```python
from build123d import *

# Parameters (mm, degrees)
BOSS_EXTRUDE1_DEPTH     = 20
CUT_EXTRUDE1_DEPTH      = 97.932966679
CUT_EXTRUDE1_DEPTH_BACK = 97.932966679
CUT_EXTRUDE3_DEPTH      = 97.932966679


with BuildPart() as part:
    # Sketch2 → Boss-Extrude1 (new body)
    with BuildSketch(Plane.XY):
        Polygon((16, 16), (16, -16), (-16, -16), (-16, -11), (-11, -11), (11, -11), (11, 11), (-11, 11), (-11, 9), (-16, 14), (-16, 16), align=None)
    extrude(amount=BOSS_EXTRUDE1_DEPTH)

    # Sketch3 → Loft1 section 0
    with BuildSketch(Plane.XZ.offset(16)):
        with BuildLine():
            Line((-16, 0), (16, 0))
            Line((16, 0), (16, 20))
            Line((16, 20), (-16, 20))
            Line((-16, 20), (-16, 0))
        make_face()
    # Sketch4 → Loft1 section 1
    with BuildSketch(Plane(origin=(0, -86, 0), x_dir=(-1, 0, 0), z_dir=(0, -1, 0))):
        with BuildLine():
            Line((40, 0), (-40, 0))
            Line((-40, 0), (-40, -20))
            Line((-40, -20), (40, -20))
            Line((40, -20), (40, 0))
        make_face()
    loft()

    # Sketch5 → Cut-Extrude1 (cut, two sides: drawn at the far end of the back side and taken through both)
    with BuildSketch(Plane(origin=(0, 0, 0), x_dir=(0, 0, -1), z_dir=(1, 0, 0)).offset(-CUT_EXTRUDE1_DEPTH_BACK)):
        Polygon((0, -81), (-15, -81), (-15, -64), (0, -21), align=None)
    extrude(amount=CUT_EXTRUDE1_DEPTH + CUT_EXTRUDE1_DEPTH_BACK, mode=Mode.SUBTRACT)

    # Sketch6 → Cut-Extrude3 (cut, through all)
    with BuildSketch(Plane.XY):
        Polygon((-1.810810811, -20.864864865), (1.810810811, -20.864864865), (19, -71), (-19, -71), align=None)
    extrude(amount=CUT_EXTRUDE3_DEPTH, mode=Mode.SUBTRACT)


solid = part.part
```
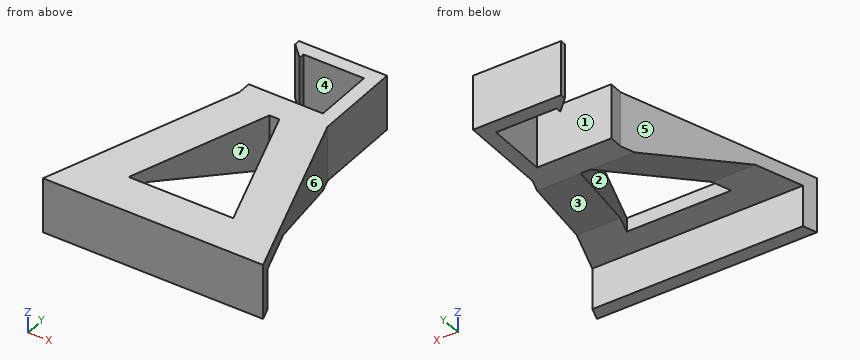
Design review of the part built by this model. Coordinates are the model's own, in mm. Face numbers are marked on the shaded views. A direction names the side the tool comes from. Give positions to 0.01 mm unless a question says otherwise; leave off trailing zeros. Write each loop counter-clockwise with the first axis right and the second up, starting at its lowest first coordinate (ties: lowest second). Pieces come first, ordered by that corner, then holes. Notation, with made-up numbers: (-34.5, -2) -> (-2.5, -2) arc R19 ccw to (-2.5, 8) -> close; hole circle Ø2 at (-39, 20.5). An arc over 180 degrees is marked (long way). Answer in a Markdown table with one row per item.
(1) Mouldability with a two-part tool opening along X and no side actions: class the marked faces 4, 5, 6 and 7 as +X half, -X half, draft (parallel to the pull), parting line (faces both ways), or undercut.
Results:
| item | result |
|---|---|
| face 4 | undercut |
| face 5 | -X half |
| face 6 | +X half |
| face 7 | undercut |
(2) Consider section A-A (z = 13.5). State the section outline as (x, y) points.
Results:
| item | result |
|---|---|
| outline | (-40, -86) -> (40, -86) -> (38.29, -81) -> (-38.29, -81) -> close; (-30.98, -59.7) -> (-15.13, -59.7) -> (-1.81, -20.86) -> (1.81, -20.86) -> (15.13, -59.7) -> (30.98, -59.7) -> (16, -16) -> (16, 16) -> (-16, 16) -> (-16, 14) -> (-11, 9) -> (-11, 11) -> (11, 11) -> (11, -11) -> (-16, -11) -> (-16, -16) -> close |
(3) Consider section D-D (x = -6.5). State the section outline as (y, z) points, then the cut area to 3 significant figures.
Results:
| item | result |
|---|---|
| outline | (-86, 0) -> (-81, 0) -> (-81, 15) -> (-71, 15) -> (-71, 20) -> (-86, 20) -> close; (-34.54, 4.72) -> (-21, 0) -> (-11, 0) -> (-11, 20) -> (-34.54, 20) -> close; (11, 0) -> (16, 0) -> (16, 20) -> (11, 20) -> close |
| area | 689 mm2 |
(4) For the marked faces 1, 2 and 3, list the 3-axis set-ups (+Z, -Z, +X, -X, +Y, -Y) from which the entire face can be reached by the end or side of a thin tool; tool diameter is ignored.
Results:
| item | result |
|---|---|
| face 1 | +Z, -Z, -X |
| face 2 | +Z, -Z |
| face 3 | -Z, +X, -X |
(5) Consider section B-B (y = -26.5). State the section outline as (x, z) points.
Results:
| item | result |
|---|---|
| outline | (-19.6, 1.92) -> (-3.74, 1.92) -> (-3.74, 20) -> (-19.6, 20) -> close; (3.74, 1.92) -> (19.6, 1.92) -> (19.6, 20) -> (3.74, 20) -> close |
(6) Clearance check with flat-ended pins moving along their axes: pin 1 (12 mm diameter, centred on y = -12.5, z = 11, fed in from -X); pin 2 (0.6 mm diameter, centred on y = 10, z = 10.5, fed in from +X); pin 3 (1.5 mm diameter, centred on y = -19, z = 17, fed in from -X). State where each tip first meets the part, or that it passes through.
Results:
| item | result |
|---|---|
| pin 1 | x = -16.86 |
| pin 2 | x = 16 |
| pin 3 | x = -17.29 |
(7) Consider section C-C (x = -27). State the section outline as (y, z) points.
Results:
| item | result |
|---|---|
| outline | (-86, 0) -> (-81, 0) -> (-81, 15) -> (-64, 15) -> (-48.08, 9.45) -> (-48.08, 20) -> (-86, 20) -> close |
(8) To check wall thickness, follow probe 1 along X at (y, z) = (4, 8.5); probe 2 along Y at (x, z) = (-31, 3.25); probe 3 along X at (y, z) = (-31.5, 17). State the ranges of each line that lie inside material, in increasing order.
Results:
| item | result |
|---|---|
| probe 1 | 11 to 16 |
| probe 2 | -86 to -81 |
| probe 3 | -21.31 to -5.46, 5.46 to 21.31 |
